```python
from build123d import *

# Parameters (mm, degrees)
F0_W      = 31.75
F0_H      = 9.525
F1_DEPTH  = 3.175
F4_R      = 2.286
F8_R      = 2.286
F11_DEPTH = 3.175
F13_DEPTH = 52.79898
F15_DEPTH = 25.4
F17_DEPTH = 2


with BuildPart() as f1:
    # F0 (on Top) → F1 (new body)
    with BuildSketch(Plane.XY):
        with Locations((15.875, 4.7625)):
            Rectangle(F0_W, F0_H)
    extrude(amount=F1_DEPTH)

    # F5: sweep along a path in F3
    with BuildLine(Plane.YZ.offset(28.575)) as f5_path:
        Line((7.1374, 3.175), (7.1374, 9.525))
        Line((7.1374, 9.525), (11.6275280605, 14.0151280605))
    # F4 (on face) → F5 (sweep)
    with BuildSketch(Plane.XY.offset(3.175)):
        with Locations((28.575, 7.1374)):
            Circle(F4_R)
    sweep(path=f5_path.line, transition=Transition.RIGHT)

    # F9: sweep along a path in F7
    with BuildLine(Plane.YZ.offset(3.175)) as f9_path:
        Line((7.1374, 3.175), (7.1374, 9.525))
        Line((7.1374, 9.525), (11.6275280605, 14.0151280605))
    # F8 (on face) → F9 (sweep)
    with BuildSketch(Plane.XY.offset(3.175)):
        with Locations((3.175, 7.1374)):
            Circle(F8_R)
    sweep(path=f9_path.line, transition=Transition.RIGHT)

    # F10 (on face) → F11 (join, through all)
    with BuildSketch(Plane.XY.offset(3.175)):
        with BuildLine():
            Line((32.2702801376, -4.5202594941), (41.275, 4.4844603683))
            ThreePointArc((41.275, 4.4844603683), (15.875, 12.4564875628), (-9.525, 4.4844603683))
            Line((-9.525, 4.4844603683), (-0.5202801376, -4.5202594941))
            ThreePointArc((-0.5202801376, -4.5202594941), (15.875, 0), (32.2702801376, -4.5202594941))
        make_face()
    extrude(amount=-F11_DEPTH)

    # F12 (on face) → F13 (join)
    with BuildSketch(Plane(origin=(0, 0, 0), x_dir=(1, 0, 0), z_dir=(0, 0, -1))):
        with BuildLine():
            Line((-0.5202801376, 4.5202594941), (-1.9761626677, 3.064376964))
            ThreePointArc((-1.9761626677, 3.064376964), (15.875, -2), (33.7261626677, 3.064376964))
            Line((33.7261626677, 3.064376964), (32.2702801376, 4.5202594941))
            ThreePointArc((32.2702801376, 4.5202594941), (15.875, 0), (-0.5202801376, 4.5202594941))
        make_face()
    extrude(amount=F13_DEPTH)

    # F14 (on face) → F15 (cut)
    with BuildSketch(Plane(origin=(0, 12.8213280605, 12.8213280605), x_dir=(1, 0, 0), z_dir=(0, 0.7071067812, 0.7071067812))):
        Polygon((3.175, -3.9742881508), (-2.5950474281, -3.9742881508), (-2.5950474281, -10.2548293379), (34.3450474281, -10.2548293379), (34.3450474281, -3.9742881508), align=None)
    extrude(amount=-F15_DEPTH, mode=Mode.SUBTRACT)

    # F16 (on face) → F17 (join)
    with BuildSketch(Plane(origin=(0, 0, -52.79898), x_dir=(1, 0, 0), z_dir=(0, 0, -1))):
        with BuildLine():
            ThreePointArc((19.0465359344, -1.8517272227), (15.875, -2), (12.7034640656, -1.8517272227))
            ThreePointArc((12.7034640656, -1.8517272227), (15.875, -5.175), (19.0465359344, -1.8517272227))
        make_face()
    extrude(amount=-F17_DEPTH)


solid = f1.part
```
Here's how the part is built. I have some questions about the finished solid (model axes, mm). A direction names the side the tool comes from. Coordinates: 2 decimals unless noted, no trailing zeros. Order: outer loops, then holes, each group sorted by start corner. A loop starts at its lowest first (then second) coordinate and runs counter-clockwise, first axis right, second up.
1) Imagine slicing it at B-B on z = -7. List the corners of the cut face in (x, y) for me (3 decimals).
2) We'd pull the mould along Z, two halves only. Please class faces 4 (the face through (28.1, 4.9, 6.1)), 5 (the face through (31.29, -3.01, 2.61)), 6 (the face through (16, 0, -24)): +Z half, -Z half, draft (parallel to the pull), parting line (faces both ways), or undercut.
3) Imagine slicing it at C-C on x = 2. List the corners of the cut face in (y, z) for me (1 decimal), and give its area (4 significant figures).
4) Imagine slicing it at D-D on x = 36. List the corners of the cut face in (y, z) for me (3 decimals), and give its area (3 significant figures).
5) I need wall thicknesses on line 1 (Z direction, x = 30, y = 7.5); line 2 (Z direction, x = 34.5, y = -1.25) (3 decimals); line 3 (X direction, y = 10.5, z = 12). Which ranges of each line are inside material? Lowest first, please.
6) Which directions (+Z, -Z, +X, -X, +Y, -Y) give clear straight access to the entire face, cutting with the end or side of a thin tool? Please do faces 1 (the face through (2.7, 4.9, 6.1)), 2 (the face through (16.254, 12.455, 1.61)), 3 (the face through (-0.14, -3.01, 2.61)).
7) Will these pins go through, and if not, where does the flat tip stop? pin 1 (10 mm diameter, centred on y = 3, z = 8.5, fed in from -X); pin 2 (1.5 mm diameter, centred on x = 16, z = -33.5, fed in from +Y); pin 3 (8 mm diameter, centred on x = -2.5, y = 6, fed in from -Z).
8) Imagine slicing it at A-A on x = 30. List the corners of the cut face in (y, z) for me (1 decimal).
Response values:
1. outline: (-1.976, -3.064) - (-0.52, -4.52) arc R31.994 cw to (32.27, -4.52) - (33.726, -3.064) arc R33.994 ccw to start
2. face 4: undercut
2. face 5: +Z half
2. face 6: draft
3. outline: (-3.2, -52.8) - (-1, -52.8) - (-1, 0) - (10.2, 0) - (10.2, 3.2) - (9.1, 3.2) - (9.1, 8.7) - (13, 12.6) - (10.2, 15.4) - (5.2, 10.3) - (5.2, 3.2) - (-2.4, 3.2) - (-3.2, 2.5) - close
3. area: 208.5 mm2
4. outline: (-0.791, 0) - (7.64, 0) - (7.64, 3.175) - (-0.791, 3.175) - close
4. area: 26.8 mm2
5. line 1: z = 0 to 12.42
5. line 2: z = 0 to 3.175
5. line 3: x = 0.98 to 5.37, 26.38 to 30.77
6. face 1: none
6. face 2: -Z, +Y
6. face 3: +Z, +X, -X, -Y
7. pin 1: stops at x = 0.89
7. pin 2: stops at y = 2
7. pin 3: stops at z = 0
8. outline: (-3.3, -52.8) - (-1.1, -52.8) - (-1.1, 0) - (10.2, 0) - (10.2, 3.2) - (8.9, 3.2) - (8.9, 8.8) - (12.9, 12.8) - (10.4, 15.3) - (5.3, 10.3) - (5.3, 3.2) - (-2.4, 3.2) - (-3.3, 2.3) - close
